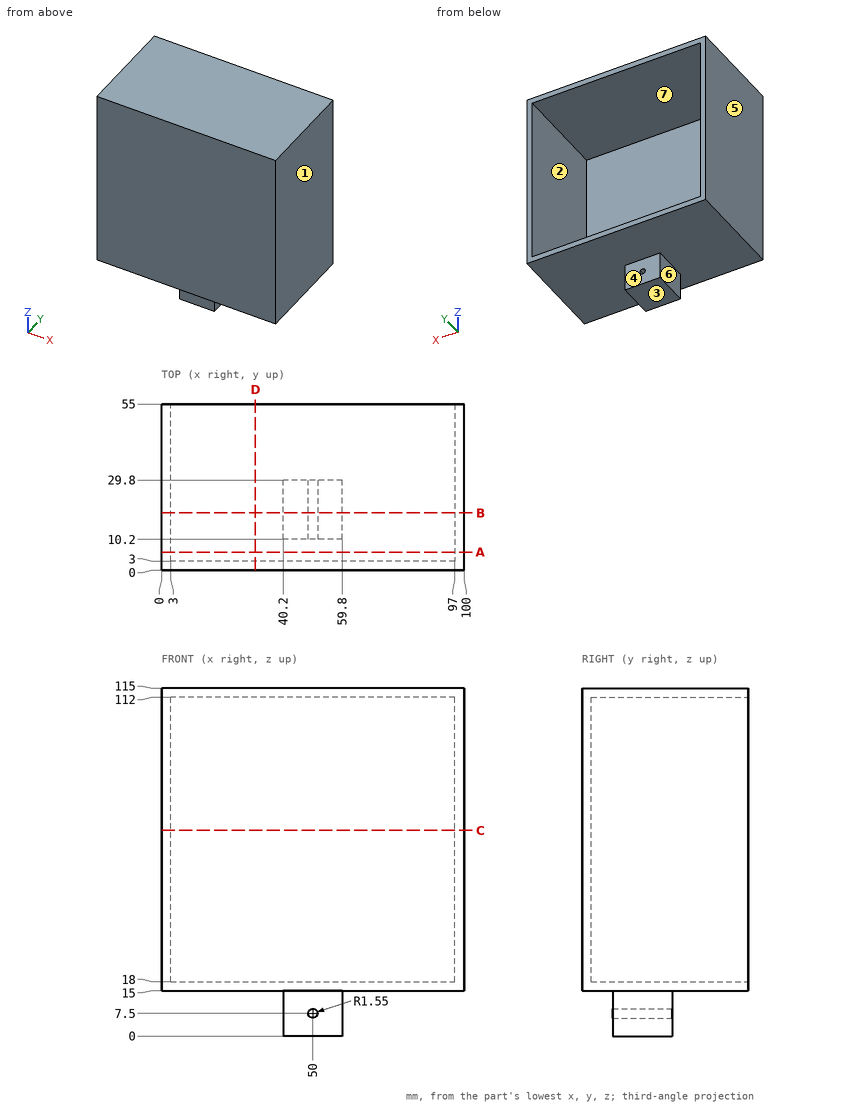
Check sheet for the drawn part. Datum: minimum x, y, z corner. Units: mm. A direction names the side the tool comes from. Round coordinates to 2 decimals unless told otherwise and drop trailing zeros. Order: outer loops, then holes, each group sorted by start corner. A loop starts at its lowest first (then second) coordinate and runs counter-clockwise, first axis right, second up.
1) Scan lines: line 1 (Z direction, x = 50, y = 16.5); line 2 (X direction, y = 34, z = 46); line 3 (Z direction, x = 7, y = 17). Record each from-to range of solid material in increasing order.
2) Mould release check, pull along Z, two halves, no side actions. Record for the marked faces 1, 2 and 3: +Z half, -Z half, draft (parallel to the pull), parting line (faces both ways), or undercut.
3) Section check A-A (y = 6). Record the boundary of the cut face in (x, z).
4) Section check D-D (x = 31). Record the boundary of the cut face in (y, z).
5) Section check B-B (y = 19). Record the boundary of the cut face in (x, z).
6) Go/stop test with flat-tipped pins: pin 1 Ø16.5 at (y, z) = (22.5, 6) entering from -X; pin 2 Ø4 at (x, z) = (65, 45.5) entering from +Y; pin 3 Ø4 at (x, y) = (14, 9) entering from -Z; pin 4 Ø2 at (y, z) = (18.5, 96) entering from -X. Record where each tip stops, or that it passes through.
7) Section check C-C (z = 68). Record the boundary of the cut face in (x, y).
8) Tool access check on the marked faces 4, 5, 6 and 7. Record the directions out of +Z, -Z, +X, -X, +Y, -Y that give a thin tool (end or side, any length) a straight path to the whole face; none if there is none.
Result:
1. line 1: z = 0 to 5.95, 9.05 to 18, 112 to 115
1. line 2: x = 0 to 3, 97 to 100
1. line 3: z = 15 to 18, 112 to 115
2. face 1: draft
2. face 2: undercut
2. face 3: -Z half
3. outline: (0, 15) - (100, 15) - (100, 115) - (0, 115) - close; hole (3, 18) - (97, 18) - (97, 112) - (3, 112) - close
4. outline: (0, 15) - (55, 15) - (55, 18) - (3, 18) - (3, 112) - (55, 112) - (55, 115) - (0, 115) - close
5. outline: (0, 15) - (40.2, 15) - (40.2, 0) - (59.8, 0) - (59.8, 15) - (100, 15) - (100, 115) - (0, 115) - close; hole (3, 18) - (97, 18) - (97, 112) - (3, 112) - close; hole circle Ø3.1 at (50, 7.5)
6. pin 1: stops at x = 40.2
6. pin 2: stops at y = 3
6. pin 3: stops at z = 15
6. pin 4: stops at x = 0
7. outline: (0, 0) - (100, 0) - (100, 55) - (97, 55) - (97, 3) - (3, 3) - (3, 55) - (0, 55) - close
8. face 4: -Z, +X, -X, +Y
8. face 5: +Z, -Z, -X, +Y, -Y
8. face 6: -Z, -X, +Y, -Y
8. face 7: +Y
